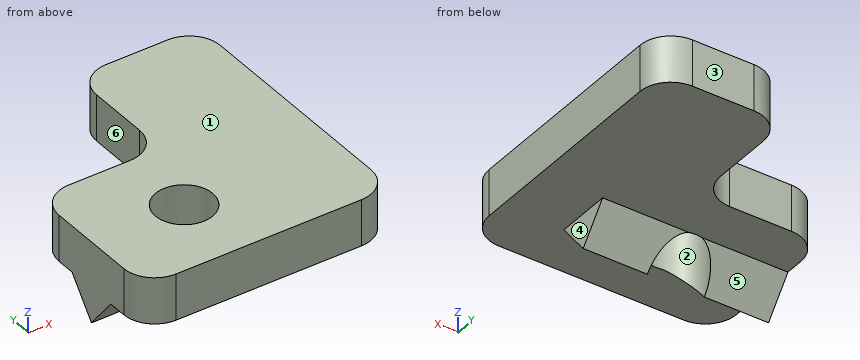
```python
from build123d import *

# Parameters (mm, degrees)
BOSS_EXTRUDE3_DEPTH = 12
SKETCH4_R           = 1.85
CUT_EXTRUDE1_DEPTH  = 12
SKETCH5_W           = 3
SKETCH5_H           = 18
BOSS_EXTRUDE4_DEPTH = 4
FILLET2_R           = 2


with BuildPart() as part:
    # Sketch3 → Boss-Extrude3 (new body)
    with BuildSketch(Plane.ZY.offset(178.52034041)):
        Polygon((-3, 14.935767061), (-5.250229512, 13.135583451), (-3, 11.335399842), (-3, 8.134419599), (0, 8.134419599), (0, 18.136747304), (-3, 18.136747304), align=None)
    extrude(amount=-BOSS_EXTRUDE3_DEPTH)

    # Sketch4 → Cut-Extrude1 (cut)
    with BuildSketch(Plane.XY):
        with Locations((-172.52034041, 13.136747304)):
            Circle(SKETCH4_R)
    extrude(amount=-CUT_EXTRUDE1_DEPTH, mode=Mode.SUBTRACT)

    # Sketch5 → Boss-Extrude4 (add, symmetric)
    with BuildSketch(Plane(origin=(-166.52034041, 0, 0), x_dir=(0, 0, -1), z_dir=(1, 0, 0))):
        with Locations((1.5, 17.134419599)):
            Rectangle(SKETCH5_W, SKETCH5_H)
    extrude(amount=BOSS_EXTRUDE4_DEPTH, both=True)

    # Fillet2
    fillet2_edges = [part.edges().sort_by_distance(p)[0] for p in [
        (-170.52034041, 18.136747304, -1.5),
        (-170.52034041, 26.134419599, -1.5),
        (-162.52034041, 8.134419599, -1.5),
        (-162.52034041, 26.134419599, -1.5),
        (-178.52034041, 18.136747304, -1.5),
        (-178.52034041, 8.134419599, -1.5),
    ]]
    fillet(fillet2_edges, radius=FILLET2_R)


solid = part.part
```
The listing builds one solid part. Answer for the finished solid, in the listing's coordinates (mm). Face numbers are marked on the shaded views. A direction names the side the tool comes from. Coordinates: 2 decimals unless noted, no trailing zeros. Loops run counter-clockwise (first coordinate to the right, second up) from the corner with the lowest first, then second, coordinate; pieces in that order, holes last. Notation, with made-up numbers: (60.25, 50.25) -> (95.25, 50.25) arc R38 cw to (95.25, 89.25) -> close; hole circle Ø1 at (5.25, 47). An arc over 180 degrees is marked (long way). Use one line per item in the form item = value. Start each with the question number.
Item 1: The part is cut by section D-D on z = -0.75. Determine the outline of the cut face in (x, y), then the cut area to 3 significant figures.
Item 2: The part is cut by section A-A on x = -173.5. Determine the outline of the cut face in (y, z).
Item 3: Flat-ended cylindrical pins translate along their axes: pin 1 Ø3 at (x, y) = (-172.52, 13.14) entering from -Z (3 decimals); pin 2 Ø2.5 at (y, z) = (13.5, -3.5) entering from +X; pin 3 Ø1.5 at (x, y) = (-166, 20.5) entering from -Z; pin 4 Ø2.5 at (x, z) = (-174.5, -1) entering from +Y. Find the tip coordinate at first contact, or state that the pin passes through.
Item 4: The part is cut by section B-B on z = -4.15. Determine the outline of the cut face in (x, y).
Item 5: Consider L1, parallel to Z at x = -166, y = 12.5; L2, parallel to X at y = 21.25, z = -1.7; L3, parallel to Y at x = -175.5, z = -0.15. Determine where each line is inside the solid, lowest interval first. Write a range as [from, to].
Item 6: The mould has two halves that part along Y. Classify the marked faces 1, 2 and 3: released by +Y, released by -Y, zero draft, split by the parting line, or undercut.
Item 7: The part is cut by section C-C on y = 12.5. Determine the outline of the cut face in (x, z).
Item 8: A tool of negligible diameter and unlimited length cuts with its end or side. For the marked faces 4, 5 and 6, from which of +Z, -Z, +X, -X, +Y, -Y can it reach the whole face along a straight path? Write none if from no direction.
Answer key:
q1.outline = (-178.52, 10.13) arc R2 ccw to (-176.52, 8.13) -> (-164.52, 8.13) arc R2 ccw to (-162.52, 10.13) -> (-162.52, 24.13) arc R2 ccw to (-164.52, 26.13) -> (-168.52, 26.13) arc R2 ccw to (-170.52, 24.13) -> (-170.52, 20.14) arc R2 cw to (-172.52, 18.14) -> (-176.52, 18.14) arc R2 ccw to (-178.52, 16.14) -> close; hole circle Ø3.7 at (-172.52, 13.14)
q1.area = 210 mm2
q2.outline = (8.13, -3) -> (11.34, -3) -> (11.57, -3.29) -> (11.57, 0) -> (8.13, 0) -> close; (14.71, -3.29) -> (14.94, -3) -> (18.14, -3) -> (18.14, 0) -> (14.71, 0) -> close
q3.pin_1 = through
q3.pin_2 = -162.52
q3.pin_3 = -3
q3.pin_4 = 18.14
q4.outline = (-178.52, 12.26) -> (-174.15, 12.26) arc R1.85 cw to (-174.15, 14.02) -> (-178.52, 14.02) -> close; (-170.89, 12.26) -> (-166.52, 12.26) -> (-166.52, 14.02) -> (-170.89, 14.02) arc R1.85 cw to start
q5.L1 = [-3, 0]
q5.L2 = [-170.52, -162.52]
q5.L3 = [8.13, 18.14]
q6.face_1 = zero draft
q6.face_2 = undercut
q6.face_3 = released by +Y
q7.outline = (-178.52, -4.46) -> (-174.26, -4.46) -> (-174.26, 0) -> (-178.52, 0) -> close; (-170.78, -4.46) -> (-166.52, -4.46) -> (-166.52, -3) -> (-162.52, -3) -> (-162.52, 0) -> (-170.78, 0) -> close
q8.face_4 = -Z, +X, +Y, -Y
q8.face_5 = -Z, +X, -X, +Y
q8.face_6 = +Z, -Z, -X, +Y
